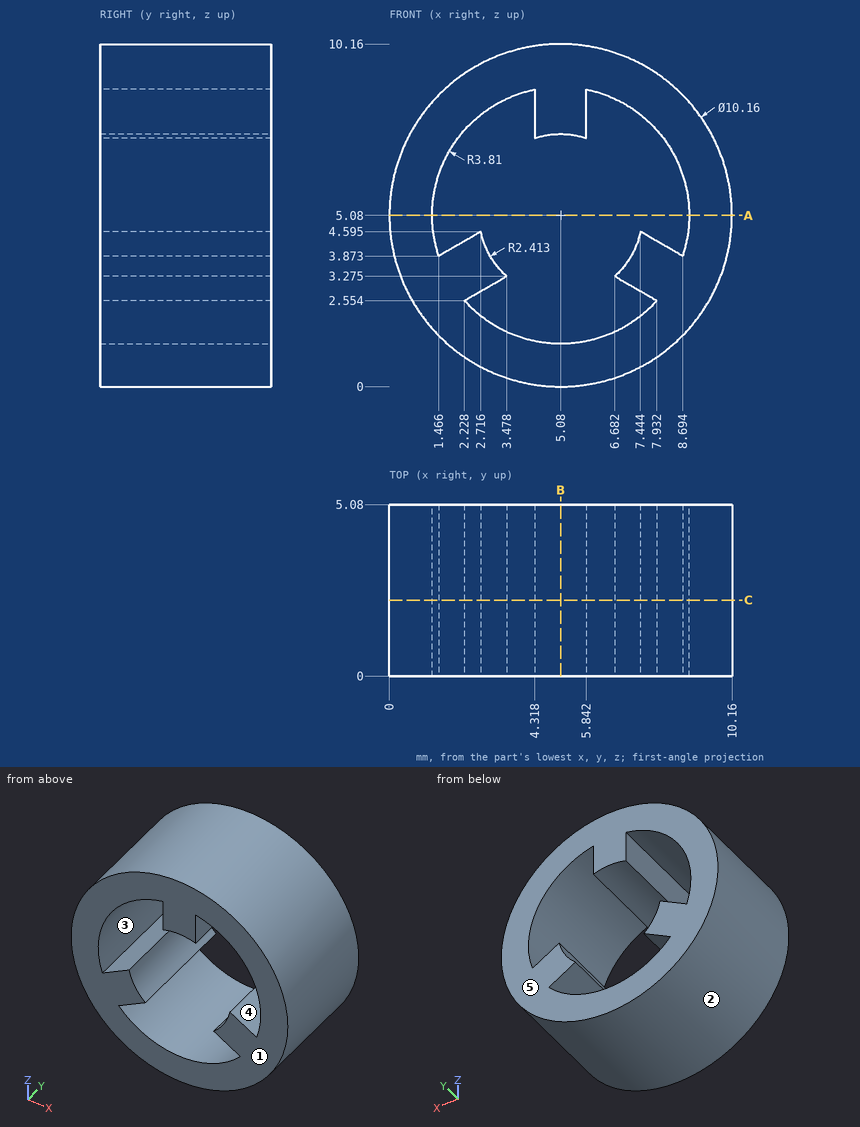
Design review of the part shown in the three views and the two pictorial views. Dimensions are in mm from the part's minimum x, y and z. A direction names the side the tool comes from. Coordinates: 2 decimals unless noted, no trailing zeros. Order: outer loops, then holes, each group sorted by start corner. A loop starts at its lowest first (then second) coordinate and runs counter-clockwise, first axis right, second up.
1) Clearance check with flat-ended pins moving along their axes: pin 1 (1.2 mm diameter, centred on y = 1.5, z = 8, fed in from +X); pin 2 (1.5 mm diameter, centred on x = 2.5, y = 0.5, fed in from -Z). State where each tip first meets the part, or that it passes through.
2) For the marked faces 4 and 5, list the 3-axis set-ups (+Z, -Z, +X, -X, +Y, -Y) from which the entire face can be reached by the end or side of a thin tool; tool diameter is ignored.
3) Take a section at B-B, the plane x = 5.08. Give the boundary of the cut face in (y, z).
4) Take a section at A-A, the plane z = 5.08. Give the boundary of the cut face in (x, y).
5) Take a section at C-C, the plane y = 2.25. Give the boundary of the cut face in (x, z) (1 decimal).
6) Mouldability with a two-part tool opening along X and no side actions: class the marked faces 1, 2 and 3 as +X half, -X half, draft (parallel to the pull), parting line (faces both ways), or undercut.
7) Wall thickness on line 1 along Z through (x, y) = (7, 4.25) (1 decimal); line 2 along Z through (x, y) = (5, 1.9); line 3 along Z through (x, y) = (3, 3.85) (1 decimal): over which ranges is each line inside the solid? List them lowest first.
Returned:
1. pin 1: stops at x = 9.6
1. pin 2: stops at z = 0.34
2. face 4: +Y, -Y
2. face 5: +Z, -Z, +X, -X, +Y
3. outline: (0, 0) - (5.08, 0) - (5.08, 1.27) - (0, 1.27) - close; (0, 7.49) - (5.08, 7.49) - (5.08, 10.16) - (0, 10.16) - close
4. outline: (0, 0) - (1.27, 0) - (1.27, 5.08) - (0, 5.08) - close; (8.89, 0) - (10.16, 0) - (10.16, 5.08) - (8.89, 5.08) - close
5. outline: circle Ø10.2 at (5.1, 5.1); hole (1.5, 3.9) - (2.7, 4.6) arc R2.4 ccw to (3.5, 3.3) - (2.2, 2.6) arc R3.8 ccw to (7.9, 2.6) - (6.7, 3.3) arc R2.4 ccw to (7.4, 4.6) - (8.7, 3.9) arc R3.8 ccw to (5.8, 8.8) - (5.8, 7.4) arc R2.4 ccw to (4.3, 7.4) - (4.3, 8.8) arc R3.8 ccw to start
6. face 1: draft
6. face 2: parting line
6. face 3: undercut
7. line 1: z = 0.4 to 1.8, 3.1 to 3.6, 8.4 to 9.8
7. line 2: z = 0 to 1.27, 7.49 to 10.16
7. line 3: z = 0.4 to 1.9, 3 to 3.9, 8.3 to 9.7
